```python
from build123d import *

# Parameters (mm, degrees)
MASTER_SKETCH_W         = 635.3556
MASTER_SKETCH_H         = 498.348
BOSS_EXTRUDE1_DEPTH     = 3.175
SKETCH2_W               = 31.75
SKETCH2_H               = 127
BOSS_EXTRUDE2_DEPTH     = 3.175
M6_CLEARANCE_HOLE1_D    = 6.6
MIRROR7_COPY_1_SKETCH_W = 31.75
MIRROR7_COPY_1_SKETCH_H = 127
MIRROR7_COPY_1_DEPTH    = 3.175
MIRROR7_COPY_2_D        = 6.6
SKETCH5_W               = 2.286
SKETCH5_H               = 69.85
CUT_EXTRUDE1_DEPTH      = 430.182420788
LPATTERN1_COUNT         = 5
LPATTERN1_PITCH         = 98.8568
SKETCH7_W               = 254
SKETCH7_H               = 2.286
CUT_EXTRUDE3_DEPTH      = 430.182420788
LPATTERN2_COUNT         = 4
LPATTERN2_PITCH         = 98.8568
MIRROR4_COPY_1_SKETCH_W = 254
MIRROR4_COPY_1_SKETCH_H = 2.286
MIRROR4_COPY_1_DEPTH    = 430.182420788
MIRROR4_COPY_2_SKETCH_W = 254
MIRROR4_COPY_2_SKETCH_H = 2.286
MIRROR4_COPY_2_DEPTH    = 430.182420788
MIRROR4_COPY_3_SKETCH_W = 254
MIRROR4_COPY_3_SKETCH_H = 2.286
MIRROR4_COPY_3_DEPTH    = 430.182420788
SKETCH10_W              = 63.5
SKETCH10_H              = 31.75
SKETCH10_R              = 3
BOSS_EXTRUDE3_DEPTH     = 3.175
M6_CLEARANCE_HOLE2_D    = 6.6
SKETCH6_W               = 254
SKETCH6_H               = 3.175
SKETCH6_W_2             = 210.6549
CUT_EXTRUDE2_DEPTH      = 449.361641774


with BuildPart() as part:
    # Master Sketch → Boss-Extrude1 (new body)
    with BuildSketch(Plane.XY):
        Rectangle(MASTER_SKETCH_W, MASTER_SKETCH_H)
    extrude(amount=BOSS_EXTRUDE1_DEPTH)

    # Sketch2 → Boss-Extrude2 (add)
    with BuildSketch(Plane.XY.offset(3.175)):
        with Locations((-333.5528, -185.674)):
            Rectangle(SKETCH2_W, SKETCH2_H)
    boss_extrude2 = extrude(amount=-BOSS_EXTRUDE2_DEPTH)

    # M6 Clearance Hole1 (through all)
    with Locations(Plane.XY.offset(3.175)):
        with Locations((-333.5528, -217.424), (-333.5528, -153.924)):
            m6_clearance_hole1 = Hole(M6_CLEARANCE_HOLE1_D / 2)

    # Mirror1: Boss-Extrude2, M6 Clearance Hole1 across plane
    add(boss_extrude2.mirror(Plane(origin=(0, 0, 0), x_dir=(0, 0, 1), z_dir=(1, 0, 0))))
    add(m6_clearance_hole1.mirror(Plane(origin=(0, 0, 0), x_dir=(0, 0, 1), z_dir=(1, 0, 0))), mode=Mode.SUBTRACT)

    # Mirror7: Boss-Extrude2, M6 Clearance Hole1 across plane
    add(boss_extrude2.mirror(Plane.ZX))
    add(m6_clearance_hole1.mirror(Plane.ZX), mode=Mode.SUBTRACT)

    # Mirror7 copy 1 sketch → Mirror7 copy 1 (add)
    with BuildSketch(Plane(origin=(0, 0, 3.175), x_dir=(-1, 0, 0), z_dir=(0, 0, 1))):
        with Locations((-333.5528, -185.674)):
            Rectangle(MIRROR7_COPY_1_SKETCH_W, MIRROR7_COPY_1_SKETCH_H)
    extrude(amount=-MIRROR7_COPY_1_DEPTH)

    # Mirror7 copy 2 (through all)
    with Locations(Plane(origin=(0, 0, 3.175), x_dir=(-1, 0, 0), z_dir=(0, 0, 1))):
        with Locations((-333.5528, -217.424), (-333.5528, -153.924)):
            Hole(MIRROR7_COPY_2_D / 2)

    # Sketch5 → Cut-Extrude1 (cut, through all)
    with BuildSketch(Plane.XY.offset(3.175)):
        with Locations((0, 197.7136)):
            Rectangle(SKETCH5_W, SKETCH5_H)
    cut_extrude1 = extrude(amount=-CUT_EXTRUDE1_DEPTH, mode=Mode.SUBTRACT)

    # LPattern1: Cut-Extrude1 ×5
    with Locations(*[(0, -i * LPATTERN1_PITCH, 0) for i in range(1, LPATTERN1_COUNT)]):
        add(cut_extrude1, mode=Mode.SUBTRACT)

    # Sketch7 → Cut-Extrude3 (cut, through all)
    with BuildSketch(Plane.XY.offset(3.175)):
        with Locations((-157.8229, 148.2852)):
            Rectangle(SKETCH7_W, SKETCH7_H)
    cut_extrude3 = extrude(amount=-CUT_EXTRUDE3_DEPTH, mode=Mode.SUBTRACT)

    # LPattern2: Cut-Extrude3 ×4
    with Locations(*[(0, -i * LPATTERN2_PITCH, 0) for i in range(1, LPATTERN2_COUNT)]):
        add(cut_extrude3, mode=Mode.SUBTRACT)

    # Mirror4: Cut-Extrude3 across plane
    add(cut_extrude3.mirror(Plane(origin=(0, 0, 0), x_dir=(0, 0, 1), z_dir=(1, 0, 0))), mode=Mode.SUBTRACT)

    # Mirror4 copy 1 sketch → Mirror4 copy 1 (cut, through all)
    with BuildSketch(Plane(origin=(0, -98.8568, 3.175), x_dir=(-1, 0, 0), z_dir=(0, 0, 1))):
        with Locations((-157.8229, -148.2852)):
            Rectangle(MIRROR4_COPY_1_SKETCH_W, MIRROR4_COPY_1_SKETCH_H)
    extrude(amount=-MIRROR4_COPY_1_DEPTH, mode=Mode.SUBTRACT)

    # Mirror4 copy 2 sketch → Mirror4 copy 2 (cut, through all)
    with BuildSketch(Plane(origin=(0, -197.7136, 3.175), x_dir=(-1, 0, 0), z_dir=(0, 0, 1))):
        with Locations((-157.8229, -148.2852)):
            Rectangle(MIRROR4_COPY_2_SKETCH_W, MIRROR4_COPY_2_SKETCH_H)
    extrude(amount=-MIRROR4_COPY_2_DEPTH, mode=Mode.SUBTRACT)

    # Mirror4 copy 3 sketch → Mirror4 copy 3 (cut, through all)
    with BuildSketch(Plane(origin=(0, -296.5704, 3.175), x_dir=(-1, 0, 0), z_dir=(0, 0, 1))):
        with Locations((-157.8229, -148.2852)):
            Rectangle(MIRROR4_COPY_3_SKETCH_W, MIRROR4_COPY_3_SKETCH_H)
    extrude(amount=-MIRROR4_COPY_3_DEPTH, mode=Mode.SUBTRACT)

    # Sketch10 → Boss-Extrude3 (add)
    with BuildSketch(Plane.XY.offset(3.175)):
        with Locations((-285.9278, 265.049)):
            Rectangle(SKETCH10_W, SKETCH10_H)
        with Locations((-285.9278, 265.049)):
            Circle(SKETCH10_R, mode=Mode.SUBTRACT)
    boss_extrude3 = extrude(amount=-BOSS_EXTRUDE3_DEPTH)

    # M6 Clearance Hole2 (through all)
    with Locations(Plane.XY.offset(3.175)):
        with Locations((-285.9278, 265.049)):
            m6_clearance_hole2 = Hole(M6_CLEARANCE_HOLE2_D / 2)

    # Mirror6: Boss-Extrude3, M6 Clearance Hole2 across plane
    add(boss_extrude3.mirror(Plane(origin=(0, 0, 0), x_dir=(0, 0, 1), z_dir=(1, 0, 0))))
    add(m6_clearance_hole2.mirror(Plane(origin=(0, 0, 0), x_dir=(0, 0, 1), z_dir=(1, 0, 0))), mode=Mode.SUBTRACT)

    # Sketch6 → Cut-Extrude2 (cut, through all)
    with BuildSketch(Plane.XY.offset(3.175)):
        with Locations((-157.8229, -247.5865)):
            Rectangle(SKETCH6_W, SKETCH6_H)
        with Locations((157.8229, -247.5865)):
            Rectangle(SKETCH6_W, SKETCH6_H)
        with Locations((-136.15035, 247.5865)):
            Rectangle(SKETCH6_W_2, SKETCH6_H)
        with Locations((136.15035, 247.5865)):
            Rectangle(SKETCH6_W_2, SKETCH6_H)
    extrude(amount=-CUT_EXTRUDE2_DEPTH, mode=Mode.SUBTRACT)


solid = part.part
```
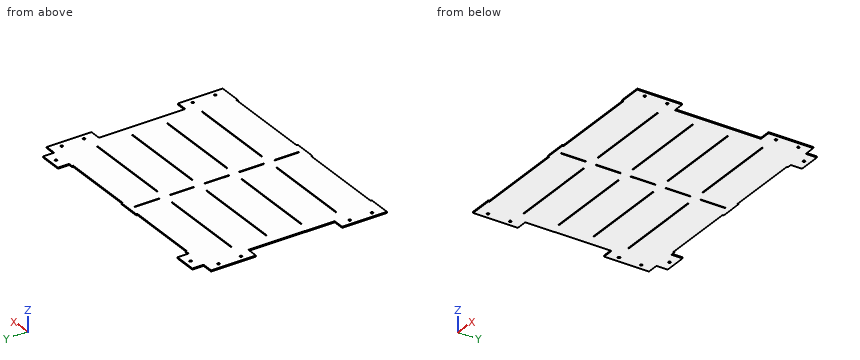
Here's how the part is built. I have some questions about the finished solid (model axes, mm). Coordinates: 2 decimals unless noted, no trailing zeros. Order: outer loops, then holes, each group sorted by start corner. A loop starts at its lowest first (then second) coordinate and runs counter-clockwise, first axis right, second up. Notation, with made-up numbers: (-32.5, 9) -> (18.5, 9) arc R16 ccw to (18.5, 14) -> close; hole circle Ø8 at (33.25, -14). An arc over 180 degrees is marked (long way). Return JSON: item names as keys, results as strings.
1) If we section it at D-D on z = 1.6: State how many separate pieces and enclosed holes the cut face has, plus the area to 3 significant figures.
Conclusion:
{"separate pieces": "1", "enclosed holes": "23", "area": "328,000 mm²"}
2) If we section it at B-B on y = 14.5: List the corners of the cut face in (x, z) for me (3 decimals).
Conclusion:
{"outline": "(-317.678, 0) -> (-1.143, 0) -> (-1.143, 3.175) -> (-317.678, 3.175) -> close; (1.143, 0) -> (317.678, 0) -> (317.678, 3.175) -> (1.143, 3.175) -> close"}
3) If I drill on probe 1 along Y at (x, z) = (127.5, 0.75); probe 2 along X at (y, z) = (-50.5, 1.3); probe 3 along X at (y, z) = (-153, 1.65), over which ranges is the centre line in solid material (lowest first)?
Conclusion:
{"probe 1": "y = -246 to -149.43, -147.14 to -50.57, -48.29 to 48.29, 50.57 to 147.14, 149.43 to 246", "probe 2": "x = -317.68 to -284.82, -30.82 to 30.82, 284.82 to 317.68", "probe 3": "x = -349.43 to -336.72, -330.38 to 330.38, 336.72 to 349.43"}
4) If we section it at A-A on x = -61: List the corners of the cut face in (y, z) for me (3 decimals).
Conclusion:
{"outline": "(-245.999, 0) -> (-149.428, 0) -> (-149.428, 3.175) -> (-245.999, 3.175) -> close; (-147.142, 0) -> (-50.571, 0) -> (-50.571, 3.175) -> (-147.142, 3.175) -> close; (-48.285, 0) -> (48.285, 0) -> (48.285, 3.175) -> (-48.285, 3.175) -> close; (50.571, 0) -> (147.142, 0) -> (147.142, 3.175) -> (50.571, 3.175) -> close; (149.428, 0) -> (245.999, 0) -> (245.999, 3.175) -> (149.428, 3.175) -> close"}
5) I'm going to push flat-ended pins straight in: P1, Ø1.8, axis at y = 49.5, z = 1, coming from the -X side; P2, Ø1, axis at x = -87.5, z = 1.5, coming from the +Y side; P3, Ø1.1, axis at x = -0.5, z = 2.5, coming from the +Y side; P4, Ø2, axis at x = -9.5, y = -106.5, coming from the -Z side. Where does each tip first touch, or does it pass through?
Conclusion:
{"P1": "stops at x = -317.68", "P2": "stops at y = 246", "P3": "stops at y = 249.17", "P4": "stops at z = 0"}
6) If we section it at C-C on x = -266.5: List the corners of the cut face in (y, z) for me (3 decimals).
Conclusion:
{"outline": "(-245.999, 0) -> (-149.428, 0) -> (-149.428, 3.175) -> (-245.999, 3.175) -> close; (-147.142, 0) -> (-50.571, 0) -> (-50.571, 3.175) -> (-147.142, 3.175) -> close; (-48.285, 0) -> (48.285, 0) -> (48.285, 3.175) -> (-48.285, 3.175) -> close; (50.571, 0) -> (147.142, 0) -> (147.142, 3.175) -> (50.571, 3.175) -> close; (149.428, 0) -> (280.924, 0) -> (280.924, 3.175) -> (149.428, 3.175) -> close"}
